Geometry check sheet. Reference: the model listing, model coordinates, mm. A direction names the side the tool comes from. Round coordinates to 2 decimals unless told otherwise and drop trailing zeros. Order: outer loops, then holes, each group sorted by start corner. A loop starts at its lowest first (then second) coordinate and runs counter-clockwise, first axis right, second up.
(1) Release check for a two-part mould opening along X. For faces 4 (the face through (33.92, 30.34, -1.01)), 5 (the face through (6, 0, -4)), 6 (the face through (31.444, 4.401, -3.397)) record: +X half, -X half, draft (parallel to the pull), parting line (faces both ways), or undercut.
(2) Material ranges on line 1 along Y through (x, z) = (-24, -2.25); line 2 along Y through (x, z) = (20.5, -2.75); line 3 along X through (y, z) = (47, -3.5), recorded low to high.
(3) Sectioned sample at A-A (x = -17). Record the boundary of the cut face in (y, z).
(4) Go/stop test with flat-tipped pins: pin 1 (1.5 mm diameter, centred on x = -15.5, z = -3.5, fed in from -Y); pin 2 (21.5 mm diameter, centred on x = 13.5, y = 23.5, fed in from +Z); pin 3 (1.7 mm diameter, centred on y = 1, z = -2.5, fed in from -X). Record where each tip stops, or that it passes through.
(5) Sectioned sample at B-B (y = 43.5). Record the boundary of the cut face in (x, z).
(6) Sectioned sample at D-D (y = 23). Record the boundary of the cut face in (x, z), plus the area to 3 significant figures.
(7) Sectioned sample at C-C (x = 4). Record the boundary of the cut face in (y, z).
(8) Set-up check for faces 1 (the face through (25.9, 28, -4)), 2 (the face through (9.77, 0.97, -1.24)), 3 (the face through (-10, 1, -3)): record each of +Z, -Z, +X, -X, +Y, -Y from which the full face is reachable in a straight line by a thin tool's end or side.
from build123d import *

# Parameters (mm, degrees)
PAD015_DEPTH         = 6
SKETCH035_W          = 80
SKETCH035_H          = 14
POCKET011_DEPTH      = 60.001
POCKET011_DEPTH_BACK = 0.001
POCKET020_DEPTH      = 5.001
POCKET021_DEPTH      = 5.001
POCKET022_DEPTH      = 5.001
SKETCH054_W          = 34
SKETCH054_H          = 43
POCKET023_DEPTH      = 4.801
SKETCH055_R          = 3.2
POCKET024_DEPTH      = 6.001
SKETCH056_W          = 11
SKETCH056_H          = 9
POCKET025_DEPTH      = 6.001
SKETCH057_W          = 10
SKETCH057_H          = 8
POCKET026_DEPTH      = 5


with BuildPart() as part:
    # Sketch033 → Pad015 (new body, symmetric)
    with BuildSketch(Plane.XY):
        with BuildLine():
            Line((29, 60), (-29, 60))
            ThreePointArc((-29, 60), (-33.242641, 58.242641), (-35, 54))
            Line((-35, 54), (-35, 6))
            ThreePointArc((-35, 6), (-33.242641, 1.757359), (-29, 0))
            Line((-29, 0), (29, 0))
            ThreePointArc((29, 0), (33.242641, 1.757359), (35, 6))
            Line((35, 6), (35, 54))
            ThreePointArc((35, 54), (33.242641, 58.242641), (29, 60))
        make_face()
    extrude(amount=PAD015_DEPTH, both=True)

    # Sketch035 → Pocket011 (cut, two sides)
    with BuildSketch(Plane.XZ) as pocket011_sk:
        with Locations((0, 5)):
            Rectangle(SKETCH035_W, SKETCH035_H)
    extrude(amount=-POCKET011_DEPTH, mode=Mode.SUBTRACT)
    extrude(pocket011_sk.sketch, amount=POCKET011_DEPTH_BACK, mode=Mode.SUBTRACT)

    # AdditivePipe: sweep along a path in Sketch033
    with BuildLine(Plane.XY) as additivepipe_path:
        Line((29, 60), (-29, 60))
        ThreePointArc((-29, 60), (-33.242641, 58.242641), (-35, 54))
        Line((-35, 54), (-35, 6))
        ThreePointArc((-35, 6), (-33.242641, 1.757359), (-29, 0))
        Line((-29, 0), (29, 0))
        ThreePointArc((29, 0), (33.242641, 1.757359), (35, 6))
        Line((35, 6), (35, 54))
        ThreePointArc((35, 54), (33.242641, 58.242641), (29, 60))
    # Sketch058 → AdditivePipe (sweep)
    with BuildSketch(Plane.XZ.offset(-30)):
        Polygon((34.382615, -2), (31.617385, -2), (32.55, 0), (33.45, 0), align=None)
    sweep(path=additivepipe_path.line)

    # Sketch050 → Pocket020 (cut, through all)
    with BuildSketch(Plane.XY.offset(-5)):
        with BuildLine():
            Line((0, 54.3), (25.1, 54.3))
            ThreePointArc((25.9, 53.5), (25.665685, 54.065685), (25.1, 54.3))
            Line((25.9, 53.5), (25.9, 2))
            ThreePointArc((25.1, 1.2), (25.665685, 1.434315), (25.9, 2))
            Line((25.1, 1.2), (0, 1.2))
            ThreePointArc((-0.8, 2), (-0.565685, 1.434315), (0, 1.2))
            Line((-0.8, 2), (-0.8, 53.5))
            ThreePointArc((0, 54.3), (-0.565685, 54.065685), (-0.8, 53.5))
        make_face()
    extrude(amount=POCKET020_DEPTH, mode=Mode.SUBTRACT)

    # Sketch052 → Pocket021 (cut, through all)
    with BuildSketch(Plane(origin=(0, -6, -5), x_dir=(1, 0, 0), z_dir=(0, 0, 1))):
        with BuildLine():
            Line((-27.8, 43.5), (-2.2, 43.5))
            ThreePointArc((-1.2, 42.5), (-1.492893, 43.207107), (-2.2, 43.5))
            Line((-1.2, 42.5), (-1.2, 8.5))
            ThreePointArc((-2.2, 7.5), (-1.492893, 7.792893), (-1.2, 8.5))
            Line((-2.2, 7.5), (-27.8, 7.5))
            ThreePointArc((-28.8, 8.5), (-28.507107, 7.792893), (-27.8, 7.5))
            Line((-28.8, 8.5), (-28.8, 42.5))
            ThreePointArc((-27.8, 43.5), (-28.507107, 43.207107), (-28.8, 42.5))
        make_face()
    extrude(amount=POCKET021_DEPTH, mode=Mode.SUBTRACT)

    # Sketch051 → Pocket022 (cut, through all)
    with BuildSketch(Plane(origin=(0, -6, -5), x_dir=(1, 0, 0), z_dir=(0, 0, 1))):
        with BuildLine():
            Line((-24.5, 63.75), (-2.5, 63.75))
            ThreePointArc((-1.5, 62.75), (-1.792893, 63.457107), (-2.5, 63.75))
            Line((-1.5, 62.75), (-1.5, 45.25))
            ThreePointArc((-2.5, 44.25), (-1.792893, 44.542893), (-1.5, 45.25))
            Line((-2.5, 44.25), (-24.5, 44.25))
            ThreePointArc((-25.5, 45.25), (-25.207107, 44.542893), (-24.5, 44.25))
            Line((-25.5, 45.25), (-25.5, 62.75))
            ThreePointArc((-24.5, 63.75), (-25.207107, 63.457107), (-25.5, 62.75))
        make_face()
    extrude(amount=POCKET022_DEPTH, mode=Mode.SUBTRACT)

    # Sketch047 → Groove002 (revolve, cut)
    with BuildSketch(Plane.XZ.offset(-55)):
        Polygon((-30, 4.5), (-29.6, 4.5), (-28.2, -5), (-27.2, -6), (-30, -6), align=None)
    revolve(axis=Axis((-30, 55, 4.5), (0, 0, 1)), mode=Mode.SUBTRACT)

    # Sketch046 → Groove003 (revolve, cut)
    with BuildSketch(Plane.XZ.offset(-5)):
        Polygon((30, 4.5), (30.4, 4.5), (31.8, -5), (32.8, -6), (30, -6), align=None)
    revolve(axis=Axis((30, 5, 4.5), (0, 0, 1)), mode=Mode.SUBTRACT)

    # Sketch054 → Pocket023 (cut, through all)
    with BuildSketch(Plane.XY.offset(-4.8)):
        with Locations((-6, 29.5)):
            Rectangle(SKETCH054_W, SKETCH054_H)
    extrude(amount=POCKET023_DEPTH, mode=Mode.SUBTRACT)

    # Sketch055 → Pocket024 (cut, through all)
    with BuildSketch(Plane.XY):
        with Locations((-4.631189, 45.448315)):
            Circle(SKETCH055_R)
    extrude(amount=-POCKET024_DEPTH, mode=Mode.SUBTRACT)

    # Sketch056 → Pocket025 (cut, through all)
    with BuildSketch(Plane.XY):
        with Locations((-15, 6.6)):
            Rectangle(SKETCH056_W, SKETCH056_H)
    extrude(amount=-POCKET025_DEPTH, mode=Mode.SUBTRACT)

    # Sketch057 → Pocket026 (cut)
    with BuildSketch(Plane.XZ):
        with Locations((-15, -1.5)):
            Rectangle(SKETCH057_W, SKETCH057_H)
    extrude(amount=-POCKET026_DEPTH, mode=Mode.SUBTRACT)

    # Sketch053 → Revolution002 (revolve)
    with BuildSketch(Plane.YZ.offset(12.3)):
        with BuildLine():
            Line((38, -1.5), (38, -5))
            Line((38, -5), (41.5, -5))
            ThreePointArc((39.5, -3), (40.085786, -4.414214), (41.5, -5))
            Line((39.5, -3), (39.5, -1.5))
            Line((39.5, -1.5), (38, -1.5))
        make_face()
    revolve(axis=Axis((12.3, 38, -1.5), (0, 0, 1)))


solid = part.part
Answer below:
1. face 4: +X half
1. face 5: draft
1. face 6: undercut
2. line 1: y = 0 to 1.5, 37.5 to 38.25, 57.75 to 60
2. line 2: y = 0 to 1.2, 54.3 to 60
2. line 3: x = -35 to -25.5, 25.9 to 35
3. outline: (0, -6) - (2.1, -6) - (2.1, -5.5) - (0, -5.5) - close; (11.1, -6) - (60, -6) - (60, -2) - (59.38, -2) - (58.45, 0) - (57.75, 0) - (57.75, -5) - (38.25, -5) - (38.25, -4.8) - (37.5, -4.8) - (37.5, -5) - (11.1, -5) - close
4. pin 1: stops at y = 57.75
4. pin 2: stops at z = -5
4. pin 3: stops at x = -33.33
5. outline: (-35, -6) - (-7.17, -6) - (-7.17, -5) - (-25.5, -5) - (-25.5, -2) - (-31.62, -2) - (-32.55, 0) - (-33.45, 0) - (-34.38, -2) - (-35, -2) - close; (-2.09, -6) - (35, -6) - (35, -2) - (34.38, -2) - (33.45, 0) - (32.55, 0) - (31.62, -2) - (25.9, -2) - (25.9, -5) - (-0.8, -5) - (-0.8, -4.8) - (-1.5, -4.8) - (-1.5, -5) - (-2.09, -5) - close
6. outline: (-35, -6) - (35, -6) - (35, -2) - (34.38, -2) - (33.45, 0) - (32.55, 0) - (31.62, -2) - (25.9, -2) - (25.9, -5) - (-0.8, -5) - (-0.8, -4.8) - (-1.2, -4.8) - (-1.2, -5) - (-28.8, -5) - (-28.8, -2) - (-31.62, -2) - (-32.55, 0) - (-33.45, 0) - (-34.38, -2) - (-35, -2) - close
6. area: 123 mm2
7. outline: (0, -6) - (60, -6) - (60, -2) - (59.38, -2) - (58.45, 0) - (57.55, 0) - (56.62, -2) - (54.3, -2) - (54.3, -5) - (1.2, -5) - (1.2, -0.75) - (0.62, -2) - (0, -2) - close
8. face 1: +Z
8. face 2: +Z, +X, -X, -Y
8. face 3: +Z, -Y
